Geometry: see drawing. Coordinates: mm, zero at the bounding-box minimum. Coordinates: 2 decimals unless noted, no trailing zeros. Write each loop counter-clockwise with the first axis right and the second up, starting at its lowest first coordinate (ties: lowest second). Pieces come first, ordered by that corner, then holes. Notation, with made-up numbers: (-5.75, 43.5) -> (40.25, 43.5) arc R19 cw to (40.25, 72.5) -> close; hole circle Ø8 at (52.5, 77). An arc over 180 degrees is marked (long way). Use one line per item in the form item = value. Start each with the question number.
(1) Cut plane A-A on z = 3.5. Return the cut outline in (x, y), plus the area to 3 significant figures.
(2) First-contact query: pin 1 (2.5 mm diameter, centred on y = 3.5, z = 3.5, fed in from +X); pin 2 (2 mm diameter, centred on x = 4, y = 6, fed in from -Z); pin 3 (2 mm diameter, centred on x = 3.5, y = 1, fed in from +Z). Flat tips, straight axial feed; report the tip coordinate or a pass-through.
(3) Ray query, line 1 along Y through (x, z) = (1.65, 3.5); line 2 along Z through (x, y) = (0.9, 2.75); line 3 along Y through (x, z) = (0.35, 3.5). Return the intervals inside material, ascending.
(4) Pull-direction query (Z, two-part tool) for the marked faces 1, 2 and 3; classes: released by +Z, released by -Z, zero draft, split by the parting line, or undercut.
(5) Cut plane B-B on x = 3.05. Return the cut outline in (y, z).
(6) Cut plane C-C on x = 4.35. Return the cut outline in (y, z).
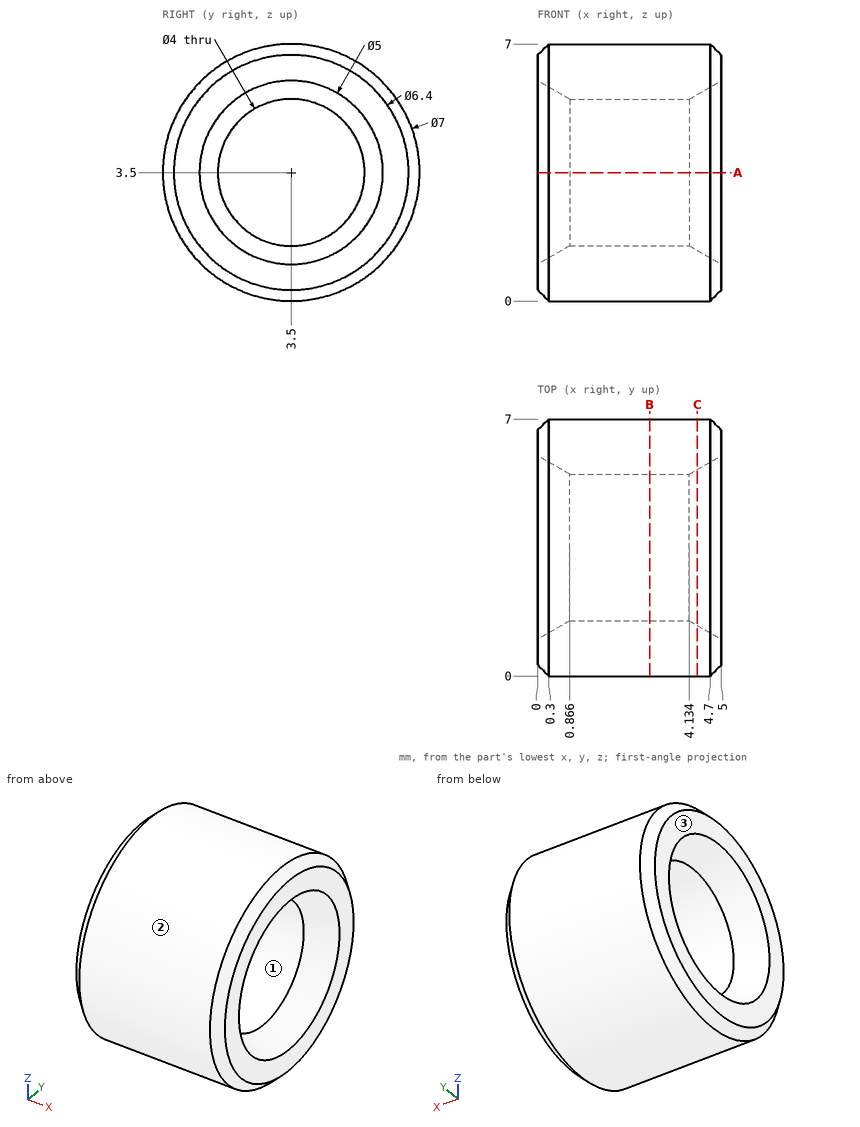
Values:
q1.outline = (0, 0.3) -> (0.3, 0) -> (4.7, 0) -> (5, 0.3) -> (5, 1) -> (4.13, 1.5) -> (0.87, 1.5) -> (0, 1) -> close; (0, 6) -> (0.87, 5.5) -> (4.13, 5.5) -> (5, 6) -> (5, 6.7) -> (4.7, 7) -> (0.3, 7) -> (0, 6.7) -> close
q1.area = 14.0 mm2
q2.pin_1 = through
q2.pin_2 = 0.34
q2.pin_3 = 6.66
q3.line_1 = 0 to 1.5, 5.5 to 7
q3.line_2 = 0.08 to 1.65, 5.35 to 6.92
q3.line_3 = 0 to 1.2, 5.8 to 7
q4.face_1 = undercut
q4.face_2 = split by the parting line
q4.face_3 = zero draft
q5.outline = circle Ø7 at (3.5, 3.5); hole circle Ø4 at (3.5, 3.5)
q6.outline = circle Ø7 at (3.5, 3.5); hole circle Ø4.25 at (3.5, 3.5)
